Could you check a few things on this model? Use its own coordinates, in mm. A direction names the side the tool comes from. Round coordinates to 2 decimals unless told otherwise and drop trailing zeros. Write each loop counter-clockwise with the first axis right and the second up, starting at its lowest first coordinate (ties: lowest second). Pieces come first, ordered by that corner, then holes. Notation, with made-up numbers: (8, 88) -> (29, 88) arc R6 ccw to (29, 94) -> close; hole circle Ø1 at (47.25, -32.75). An arc over 180 degrees is marked (long way). One line per question, with ' | ' between items. Start each with the question number.
1. For faces 1 (the cylindrical face through (2.999, 2.958, -5.767)), 2 (the flat face through (4, 4, 4)), 3 (the cylindrical face through (7.01, 1.52, -0.44)), 4 (the flat face through (-4, 4, -4)), which set-ups out of +Z, -Z, +X, -X, +Y, -Y let a thin tool reach every point of the face, with its end or its side?
2. Imagine slicing it at B-B, the plane z = 10. List the corners of the cut face in (x, y) for me.
3. Imagine slicing it at D-D, the plane x = 4.5. List the corners of the cut face in (y, z) for me, and give its area (3 significant figures).
4. Imagine slicing it at C-C, the plane x = -9.5. List the corners of the cut face in (y, z) for me, and give its area (3 significant figures).
5. If I drill on line 1 along Y through (x, z) = (3.5, 0); line 2 along X through (y, z) = (1.05, 4); line 3 along Z through (x, y) = (-8.5, 1.35), over which ranges is the centre line in solid material (lowest first)? Write a range as [from, to].
6. For pin 1 Ø5.5 at (x, z) = (-5, -3.5) entering from +Y; pin 2 Ø1.5 at (y, z) = (2, 15.5) entering from -X; pin 3 Ø3 at (y, z) = (3, -20) entering from -X; pin 4 Ø1.5 at (x, y) = (0, 1) entering from -Z, each with a flat end and sliding along its axis, tell me the tip position at first contact or that it passes through.
7. Thinking about a two-plate mould opening in X: for faces 5 (the cylindrical face through (23.37, 1.521, -0.635)), 6 (the flat face through (-3, 4, 4)), which applies, released by +X, released by -X, zero draft, split by the parting line, or undercut?
8. Imagine slicing it at A-A, the plane y = 4.95. List the corners of the cut face in (x, z) for me.
Autodesk Inventor part; units mm, degrees
ref_plane "YZ Plane" through (0, 0, 0) normal (1, 0, 0) x (0, 1, 0)
ref_plane "XZ Plane" through (0, 0, 0) normal (0, 1, 0) x (-1, 0, 0)
ref_plane "XY Plane" through (0, 0, 0) normal (0, 0, 1) x (1, 0, 0)
sketch "Sketch1" plane through (0, 0, 0) normal (0, 1, 0) x (-1, 0, 0)
  circle A0 centre (0, 0) radius 27.25
  line L0 (0, 0) -> (0, 27.25)
  line L1 (0, 0) -> (0, -27.25)
  line L2 (0, 0) -> (-27.25, 0)
  line L3 (0, 0) -> (27.25, 0)
  circle A1 centre (0, 0) radius 24
  circle A2 centre (0, 0) radius 2.55
  circle A3 centre (0, 0) radius 6.5
  point P0 (24, 0)
  point P1 (2.55, 0)
  point P2 (0, -2.55)
  point P3 (0, -24)
  point P4 (-24, 0)
  point P5 (-2.55, 0)
  point P6 (0, 2.55)
  point P7 (0, 24)
  point P8 (-6.5, 0)
  point P9 (0, -6.5)
  point P10 (6.5, 0)
  point P11 (0, 6.5)
  dimension "d0" = 54.5
  dimension "d1" = 48
  dimension "d2" = 5.1
  dimension "d5" = 13
extrude "Extrusion1" add sketch "Sketch1" along normal blind 3 contours L3 A1 L0 A0 | A0 L1 A1 L3 | L0 A1 L2 A0 | A0 L2 A1 L1 | A1 L1 A3 L3 | L0 A3 L2 A1 | A3 L1 A2 L3 | L3 A2 L0 A3 | L0 A2 L2 A3 | A3 L2 A2 L1
fillet "Fillet1" radius 2 8 edges at (-6.5, 1.5, 0) (0, 1.5, 6.5) (-24, 1.5, 0) (0, 1.5, 24) (0, 1.5, -24) (0, 1.5, -6.5) (24, 1.5, 0) (6.5, 1.5, 0)
sketch "Sketch2" plane through (0, 3, 0) normal (0, 1, 0) x (1, 0, 0)
  circle A0 centre (0, 0) radius 6.5
  dimension "d7" = 13
extrude "Extrusion2" add sketch "Sketch2" along normal blind 3
sketch "Sketch3" plane through (0, 6, 0) normal (0, 1, 0) x (1, 0, 0)
  point P0 (0, 0)
sketch "Sketch4" plane through (0, 6, 0) normal (0, 1, 0) x (1, 0, 0)
  circle A0 centre (0, 0) radius 6.5
  line L0 (5.6288, 3.2506) -> (-2.6597, -5.9309)
  line L1 (-5.6288, -3.2506) -> (2.6597, 5.9309)
  arc A1 (-1.5294, -6.3175) -> (6.3175, 1.5294) centre (0, 0) ccw
  line L2 (6.384, -1.2224) -> (-1.5727, 6.3069)
  arc A2 (1.5294, 6.3175) -> (-6.3175, -1.5294) centre (0, 0) ccw
  line L3 (-6.384, 1.2224) -> (1.5727, -6.3069)
  point P0 (-3.799, -1.2237)
  point P1 (-0.8928, -3.9737)
  point P2 (3.799, 1.2237)
  point P3 (0.8928, 3.9737)
  point P4 (-1.5727, 6.3069)
  dimension "d10" = 4
  dimension "d11" = 2
  dimension "d12" = 7
  dimension "d13" = 3.5
extrude "Extrusion3" cut sketch "Sketch4" against normal blind 2 contours A0 L3 L0 L2 | L0 L2 L1 A0 | L0 L3 L1 L2 | L0 A0 L1 L3 | L1 L3 A0 L2
sketch "Sketch5" plane through (0, 4, 0) normal (0, 1, 0) x (1, 0, 0)
  arc A0 (1.5727, -6.3069) -> (6.384, -1.2224) centre (0, 0) ccw
  line L0 (-3.799, -1.2237) -> (-6.384, 1.2224)
  line L1 (1.5727, -6.3069) -> (-6.384, 1.2224)
  arc A1 (-1.5727, 6.3069) -> (-6.384, 1.2224) centre (0, 0) ccw
  line L2 (-6.384, 1.2224) -> (-1.5727, 6.3069)
  line L3 (-1.5727, 6.3069) -> (6.384, -1.2224)
  line L4 (6.384, -1.2224) -> (1.5727, -6.3069)
extrude "Extrusion4" cut sketch "Sketch5" against normal blind 1 contours L1 L0 L2 L3 L4
sketch "Sketch7" plane through (-3.799, 4, 1.2237) normal (0.6873266, 0, -0.7263485) x (-0.7263485, 0, -0.6873266)
  line L0 (3.5589, -1) -> (3.5589, 0)
  line L1 (-7.3956, -1) -> (3.5589, -1)
  line L2 (3.5589, 0) -> (2.3243, -1)
  line L3 (-3.671, -1) -> (3.5589, -1)
  line L4 (2.3243, -1) -> (3.5589, -1)
  line L5 (3.5589, -1) -> (3.5589, 0)
  line L6 (-7.3956, 0) -> (-7.3956, 2)
  line L7 (-7.3956, -1) -> (3.5589, -1)
  line L8 (-7.3956, 0) -> (-6.161, -1)
  line L9 (-7.3956, -1) -> (-5.1497, -1)
  line L10 (-6.161, -1) -> (-7.3956, -1)
  line L11 (-7.3956, -1) -> (-7.3956, 0)
  point P0 (-1.9184, -4)
extrude "Extrusion5" add sketch "Sketch7" along normal up to next
equation "\"BendRadius\" = Thickness"
equation "\"BendReliefWidth\" = Thickness"
equation "\"BendReliefDepth\" = 0.5 * Thickness"
equation "\"CornerReliefSize\" = 4 * Thickness"
equation "\"MinimumRemnant\" = 2 * Thickness"
equation "\"TransitionRadius\" = BendRadius"
equation "\"JacobiRadiusSize\" = BendRadius"
equation "\"GapSize\" = Thickness"
properties part number "_3DPrint"
Geometry results:
1) face 1: +Y | face 2: +Z, +X, +Y | face 3: +Y, -Y | face 4: -Z, -X, +Y
2) outline: (-25.35, 0) -> (-21.82, 0) -> (-21.82, 3) -> (-25.35, 3) -> close; (0, 0) -> (25.35, 0) -> (25.35, 3) -> (0, 3) -> close
3) outline: (0, -26.88) -> (3, -26.88) -> (3, -23.57) -> (0, -23.57) -> close; (0, -4.69) -> (4, -4.69) -> (4, -2) -> (6, -2) -> (6, -0.56) -> (3, -0.56) -> (3, 1.42) -> (4, 3.21) -> (4, 4.69) -> (3, 4.69) -> (3, 26.88) -> (0, 26.88) -> close | area: 114 mm2
4) outline: (0, -25.54) -> (3, -25.54) -> (3, 0) -> (0, 0) -> close; (0, 22.04) -> (3, 22.04) -> (3, 25.54) -> (0, 25.54) -> close | area: 87.1 mm2
5) line 1: y = [0, 3] | line 2: x = [-26.95, -23.66], [-5.12, 26.95] | line 3: z = [-25.89, 0], [22.44, 25.89]
6) pin 1: stops at y = 6 | pin 2: stops at x = -22.91 | pin 3: stops at x = -20.01 | pin 4: stops at z = -27.25
7) face 5: undercut | face 6: zero draft
8) outline: (-6.38, -1.22) -> (-3.8, 1.22) -> (-5.63, 3.25) arc R6.5 ccw to start; (-2.66, 5.93) -> (-0.89, 3.97) -> (1.57, 6.31) arc R6.5 ccw to start; (-1.57, -6.31) arc R6.5 ccw to (2.66, -5.93) -> (0.89, -3.97) -> close; (3.8, -1.22) -> (5.63, -3.25) arc R6.5 ccw to (6.38, 1.22) -> close
